from build123d import *

# Parameters (mm, degrees)
SKETCH_2_W              = 145
SKETCH_2_H              = 26.443328262
SKETCH_2_W_2            = 2.5
SKETCH_2_H_2            = 2.5
EXTRUDE_1_DEPTH         = 35
EXTRUDE_1_DEPTH_BACK    = 35
SKETCH_2_4_W            = 15
SKETCH_2_4_H            = 70
CUT_EXTRUDE_1_DEPTH     = 168.493194588
HOLE_WIZARD_5_8_5_8_1_D = 5.8


with BuildPart() as part:
    # Sketch 2 → Revolve 2 (revolve)
    with BuildSketch(Plane(origin=(0, 0, 0), x_dir=(0, 0, -1), z_dir=(1, 0, 0)), mode=Mode.PRIVATE) as revolve_2_sk:
        with Locations((-72.5, -13.278335869)):
            Rectangle(SKETCH_2_W, SKETCH_2_H)
        with Locations((-161.25, -28.806671738)):
            Rectangle(SKETCH_2_W_2, SKETCH_2_H_2)
    revolve(revolve_2_sk.sketch.rotate(Axis((0, -0.056671738, 165.890142235), (0, 0, -1)), 270), axis=Axis((0, -0.056671738, 165.890142235), (0, 0, -1)))

    # Sketch 2_4 → Extrude 1 (add, two sides: drawn at the far end of the back side and taken through both)
    with BuildSketch(Plane(origin=(0, 0, 0), x_dir=(0, 0, -1), z_dir=(1, 0, 0)).offset(-EXTRUDE_1_DEPTH_BACK)):
        with Locations((-152.5, -0.056671738)):
            Rectangle(SKETCH_2_4_W, SKETCH_2_4_H)
    extrude(amount=EXTRUDE_1_DEPTH + EXTRUDE_1_DEPTH_BACK)

    # Sketch 4 → Cut-Extrude 1 (cut, through all)
    with BuildSketch(Plane.XY.offset(160)):
        with BuildLine():
            Line((-35, -35.056671738), (-25.831182706, -35.056671738))
            ThreePointArc((-25.831182706, -35.056671738), (-28.374504573, -33.028439816), (-30.759144982, -30.815816719))
            ThreePointArc((-30.759144982, -30.815816719), (-32.971768079, -28.431176311), (-35, -25.887854444))
            Line((-35, -25.887854444), (-35, -35.056671738))
        make_face()
        with BuildLine():
            ThreePointArc((35, -25.887854444), (32.971768079, -28.431176311), (30.759144982, -30.815816719))
            ThreePointArc((30.759144982, -30.815816719), (28.374504573, -33.028439816), (25.831182706, -35.056671738))
            Line((25.831182706, -35.056671738), (35, -35.056671738))
            Line((35, -35.056671738), (35, -25.887854444))
        make_face()
        with BuildLine():
            ThreePointArc((30.759144982, 30.702473244), (32.971768079, 28.317832835), (35, 25.774510968))
            Line((35, 25.774510968), (35, 34.943328262))
            Line((35, 34.943328262), (25.831182706, 34.943328262))
            ThreePointArc((25.831182706, 34.943328262), (28.374504573, 32.915096341), (30.759144982, 30.702473244))
        make_face()
        with BuildLine():
            ThreePointArc((-35, 25.774510968), (-32.971768079, 28.317832835), (-30.759144982, 30.702473244))
            ThreePointArc((-30.759144982, 30.702473244), (-28.374504573, 32.915096341), (-25.831182706, 34.943328262))
            Line((-25.831182706, 34.943328262), (-35, 34.943328262))
            Line((-35, 34.943328262), (-35, 25.774510968))
        make_face()
    extrude(amount=-CUT_EXTRUDE_1_DEPTH, mode=Mode.SUBTRACT)

    # Hole Wizard 5.8 _5.8_1 (through all)
    with Locations(Plane(origin=(-26.516504294, -26.573176032, 160), x_dir=(0, 1, 0), z_dir=(0, 0, 1))):
        with Locations((0, 0), (0, -53.033008588), (53.033008589, -53.033008588), (53.033008589, 0)):
            Hole(HOLE_WIZARD_5_8_5_8_1_D / 2)


solid = part.part
The listing builds one solid part. Answer for the finished solid, in the listing's coordinates (mm). A direction names the side the tool comes from. Coordinates: 2 decimals unless noted, no trailing zeros. Write each loop counter-clockwise with the first axis right and the second up, starting at its lowest first coordinate (ties: lowest second). Pieces come first, ordered by that corner, then holes. Notation, with made-up numbers: (7, 60) - (33, 60) arc R14 cw to (33, 82) - close; hole circle Ø9 at (-8, 85). An arc over 180 degrees is marked (long way). Put each result on its own line as item: value.
1. Flat-ended cylindrical pins translate along their axes: pin 1 Ø8 at (x, y) = (-17, 10.5) entering from -Z; pin 2 Ø4 at (y, z) = (8, 25.5) entering from +X; pin 3 Ø8 at (x, z) = (11, 97.5) entering from -Y; pin 4 Ø1.5 at (x, y) = (23, 25.5) entering from -Z. Find the tip coordinate at first contact, or state that the pin passes through.
Answer sheet:
pin 1: stops at z = 0
pin 2: stops at x = 25.74
pin 3: stops at y = -25.56
pin 4: stops at z = 145
2. The part is cut by section B-B on y = 2.5. Give the vertices of the cut face in (x, z).
Answer sheet:
outline: (-35, 145) - (-26.32, 145) - (-26.32, 0) - (26.32, 0) - (26.32, 145) - (35, 145) - (35, 160) - (29.89, 160) - (29.89, 162.5) - (27.38, 162.5) - (27.38, 160) - (-27.38, 160) - (-27.38, 162.5) - (-29.89, 162.5) - (-29.89, 160) - (-35, 160) - close
3. Determine the mould class of faces 4 (the face through (0, 34.943, 153)), 5 (the face through (0, 31, 160)), 6 (the face through (25.4, 10.48, 161.23)) for opening direction Y: pulls with the +Y half, pulls with the -Y half, needs draft (parallel to the pull), parting line crosses it, or undercut.
Answer sheet:
face 4: pulls with the +Y half
face 5: needs draft
face 6: undercut
4. A tool of negligible diameter and unlimited length cuts with its end or side. For faces 1 (the face through (-6.5, 29.23, 161.23)), 2 (the face through (23, 15, 145)), 3 (the face through (-23.685, 27.088, 152.395)), from which of +Z, -Z, +X, -X, +Y, -Y can it reach the whole face along a straight path? Write none if from no direction.
Answer sheet:
face 1: +Z
face 2: -Z
face 3: +Z, -Z
5. Find the intervals of material crossed by line 1 along X through (y, z) = (-0.5, 59); line 2 along Z through (x, y) = (-18, -6); line 3 along Y through (x, z) = (0, 161), in increasing order. Write a range as from..to.
Answer sheet:
line 1: x = -26.44..26.44
line 2: z = 0..160
line 3: y = -30.06..-27.56, 27.44..29.94
6. The part is cut by section A-A on x = 0. Give the vertices of the cut face in (y, z).
Answer sheet:
outline: (-35.06, 145) - (-26.5, 145) - (-26.5, 0) - (26.39, 0) - (26.39, 145) - (34.94, 145) - (34.94, 160) - (29.94, 160) - (29.94, 162.5) - (27.44, 162.5) - (27.44, 160) - (-27.56, 160) - (-27.56, 162.5) - (-30.06, 162.5) - (-30.06, 160) - (-35.06, 160) - close
7. The part is cut by section C-C on z = 30.5. Give the vertices of the cut face in (x, y), plus the area to 3 significant figures.
Answer sheet:
outline: circle Ø52.89 at (0, -0.06)
area: 2,200 mm^2
